The listing builds one solid part. Answer for the finished solid, in the listing's coordinates (mm). Face numbers are marked on the shaded views. A direction names the side the tool comes from. Coordinates: 2 decimals unless noted, no trailing zeros. Loops run counter-clockwise (first coordinate to the right, second up) from the corner with the lowest first, then second, coordinate; pieces in that order, holes last. Notation, with made-up numbers: (20, 7) - (72, 7) arc R19 ccw to (72, 13) - close; hole circle Ø5 at (-3, 55.25). An arc over 180 degrees is marked (long way). One line per question, with ' | ' between items.
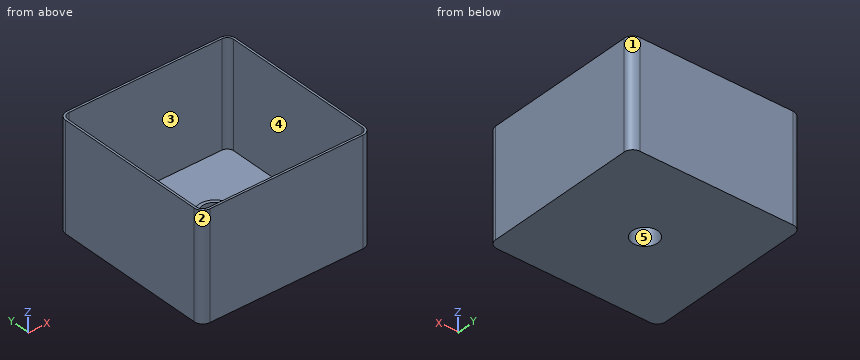
from build123d import *

# Parameters (mm, degrees)
F1_DEPTH = 50
F2_T     = -1
F3_R     = 6
F4_DEPTH = 1
F3_R_2   = 7.5
F6_DEPTH = 10


with BuildPart() as f1:
    # F0 (on Top) → F1 (new body)
    with BuildSketch(Plane.XY):
        with BuildLine():
            Line((57.163118, 69.629326), (-14.836882, 69.629326))
            ThreePointArc((-14.836882, 69.629326), (-17.665309, 68.457753), (-18.836882, 65.629326))
            Line((-18.836882, 65.629326), (-18.836882, -6.370674))
            ThreePointArc((-18.836882, -6.370674), (-17.665309, -9.199101), (-14.836882, -10.370674))
            Line((-14.836882, -10.370674), (57.163118, -10.370674))
            ThreePointArc((57.163118, -10.370674), (59.991545, -9.199101), (61.163118, -6.370674))
            Line((61.163118, -6.370674), (61.163118, 65.629326))
            ThreePointArc((61.163118, 65.629326), (59.991545, 68.457753), (57.163118, 69.629326))
        make_face()
    extrude(amount=F1_DEPTH)

    # F2
    f2_openings = [f1.faces().sort_by_distance(p)[0] for p in [
        (21.163118, 29.629326, 50),
    ]]
    offset(amount=F2_T, openings=f2_openings)

    # F3 (on face) → F4 (cut, through all)
    with BuildSketch(Plane.XY.offset(1)):
        with Locations((21.163118, 29.629326)):
            Circle(F3_R)
    extrude(amount=-F4_DEPTH, mode=Mode.SUBTRACT)

    # F3 (on face) → F6 (join)
    with BuildSketch(Plane.XY.offset(1)):
        with Locations((21.163118, 29.629326)):
            Circle(F3_R_2)
        with Locations((21.163118, 29.629326)):
            Circle(F3_R, mode=Mode.SUBTRACT)
    extrude(amount=F6_DEPTH)


solid = f1.part
Item 1: Each of these flat-tipped pins is pushed along its axis until it touches: pin 1 Ø11 at (x, y) = (21.16, 29.63) entering from +Z; pin 2 Ø16.5 at (x, y) = (24.5, 29.5) entering from +Z. Where does it stop, or does it pass through?
Taken from the geometry:
pin 1: passes through | pin 2: stops at z = 11
Item 2: Find section B-B, the plane x = 22.5. Write down the section's boundary in (y, z).
Taken from the geometry:
outline: (-10.37, 0) - (23.78, 0) - (23.78, 11) - (22.25, 11) - (22.25, 1) - (-9.37, 1) - (-9.37, 50) - (-10.37, 50) - close; (35.48, 0) - (69.63, 0) - (69.63, 50) - (68.63, 50) - (68.63, 1) - (37.01, 1) - (37.01, 11) - (35.48, 11) - close
Item 3: Find section D-D, the plane y = 5.5. Write down the section's boundary in (x, z).
Taken from the geometry:
outline: (-18.84, 0) - (61.16, 0) - (61.16, 50) - (60.16, 50) - (60.16, 1) - (-17.84, 1) - (-17.84, 50) - (-18.84, 50) - close
Item 4: The mould has two halves that part along Y. Classify the marked faces 1, 2 and 3: pulls with the +Y half, pulls with the -Y half, needs draft (parallel to the pull), parting line crosses it, or undercut.
Taken from the geometry:
face 1: pulls with the +Y half | face 2: pulls with the -Y half | face 3: undercut
Item 5: Find section C-C, the plane z = 10. Write down the section's boundary in (x, y), plus the area to 3 significant figures.
Taken from the geometry:
outline: (-18.84, -6.37) arc R4 ccw to (-14.84, -10.37) - (57.16, -10.37) arc R4 ccw to (61.16, -6.37) - (61.16, 65.63) arc R4 ccw to (57.16, 69.63) - (-14.84, 69.63) arc R4 ccw to (-18.84, 65.63) - close; circle Ø15 at (21.16, 29.63); hole (-17.84, -6.37) arc R3 ccw to (-14.84, -9.37) - (57.16, -9.37) arc R3 ccw to (60.16, -6.37) - (60.16, 65.63) arc R3 ccw to (57.16, 68.63) - (-14.84, 68.63) arc R3 ccw to (-17.84, 65.63) - close; hole circle Ø12 at (21.16, 29.63) | area: 374 mm2
Item 6: Find the intervals of material crossed by line 1 (Y direction, x = 13, z = 3.5); line 2 (X direction, y = 51.5, z = 26); line 3 (Y direction, x = 22.5, z = 9), in increasing order. Write a range as [from, to].
Taken from the geometry:
line 1: y = [-10.37, -9.37], [68.63, 69.63] | line 2: x = [-18.84, -17.84], [60.16, 61.16] | line 3: y = [-10.37, -9.37], [22.25, 23.78], [35.48, 37.01], [68.63, 69.63]
Item 7: Which of the six approach directions +Z, -Z, +X, -X, +Y, -Y give full straight-line access (tool end or side, diameter ignored) to the marked faces 4 and 5?
Taken from the geometry:
face 4: +Z | face 5: +Z, -Z
Item 8: Find section A-A, the plane z = 26.5. Write down the section's boundary in (x, y).
Taken from the geometry:
outline: (-18.84, -6.37) arc R4 ccw to (-14.84, -10.37) - (57.16, -10.37) arc R4 ccw to (61.16, -6.37) - (61.16, 65.63) arc R4 ccw to (57.16, 69.63) - (-14.84, 69.63) arc R4 ccw to (-18.84, 65.63) - close; hole (-17.84, -6.37) arc R3 ccw to (-14.84, -9.37) - (57.16, -9.37) arc R3 ccw to (60.16, -6.37) - (60.16, 65.63) arc R3 ccw to (57.16, 68.63) - (-14.84, 68.63) arc R3 ccw to (-17.84, 65.63) - close
